For this review, take the finished solid that the model builds, in its own axes (mm). Face numbers are marked on the shaded views. A direction names the side the tool comes from. Coordinates: 2 decimals unless noted, no trailing zeros. Write each loop counter-clockwise with the first axis right and the second up, starting at its lowest first coordinate (ties: lowest second). Pieces come first, ordered by that corner, then holes. Notation, with made-up numbers: (82.25, 58.5) - (141.25, 58.5) arc R10 cw to (141.25, 62.5) - close; hole circle Ø1 at (-25.5, -30). An arc over 180 degrees is marked (long way). Use one line per item in the form item = value. Start each with the question number.
1) Mouldability with a two-part tool opening along Y and no side actions: class the marked faces 1, 2, 3 and 4 as pulls with the +Y half, pulls with the -Y half, needs draft (parallel to the pull), parting line crosses it, or undercut.
2) We need section C-C (y = -20). Give the boundary of the cut face in (x, z), plus the area to 3 significant figures.
3) Tool access review of the marked faces 5, 6, 7 and 8: name each direction out of +Z, -Z, +X, -X, +Y, -Y from which nothing blocks a thin tool from reaching the whole face with its end or side.
4) Insertion check: P1, Ø3, axis at x = 9, y = 5, coming from the -Z side; P2, Ø3, axis at y = 2, z = -2, coming from the +X side; P3, Ø1, axis at y = 11.5, z = 1, coming from the -X side; P4, Ø3, axis at x = -0.84, y = -12.32, coming from the +Z side. Each pin has a flat end and moves straight along its axis. Give the tip position at first contact, or say it passes through.
5) We need section A-A (z = 1). Count the separate pieces of the cut face and the enclosed holes in it, plus the area to 3 significant figures.
6) For L1, parallel to Y at x = -1.5, z = -3.75; L2, parallel to Y at x = 1, z = -1.5; L3, parallel to Z at x = 12.5, y = -3.5, list the stretches that pass through material, from the lowest coordinate up. Write a range as from..to.
7) We need section D-D (x = 12). Give the boundary of the cut face in (y, z).
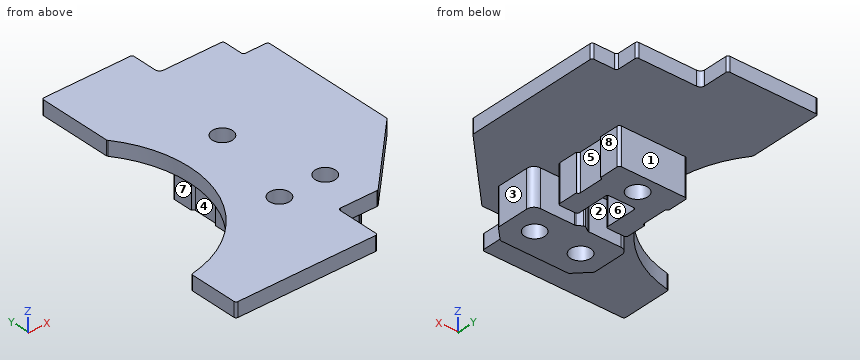
Autodesk Inventor part; units mm, degrees
ref_plane "Work Plane1" through (-17.3538, -25.3153, -5.1) normal (0, 0, 1) x (1, 0, 0)
ref_plane "Work Plane2" through (282.7327, 0, 0) normal (0, 0, 1) x (1, 0, 0)
ref_plane "YZ Plane" through (0, 0, 0) normal (1, 0, 0) x (0, 1, 0)
ref_plane "Work Plane1" through (-17.3538, -25.3153, -5.1) normal (0, 0, 1) x (1, 0, 0)
sketch "holes" plane through (0, 0, 0) normal (0, 0, 1) x (1, 0, 0)
  arc A0 (17.3538, 10.1647) -> (17.0538, 10.4647) centre (17.0538, 10.1647) ccw
  line L0 (17.0538, 10.4647) -> (14.2323, 10.4647)
  arc A1 (13.9323, 10.7647) -> (14.2323, 10.4647) centre (14.2323, 10.7647) ccw
  line L1 (13.9323, 10.7647) -> (13.9323, 13.3588)
  arc A2 (13.9323, 13.3588) -> (13.6323, 13.6588) centre (13.6323, 13.3588) ccw
  line L2 (13.6323, 13.6588) -> (5.6606, 13.6588)
  arc A3 (5.0636, 14.2558) -> (5.6606, 13.6588) centre (5.6606, 14.2558) ccw
  line L3 (5.0636, 14.2558) -> (5.0636, 17.6129)
  arc A4 (5.0636, 17.6129) -> (4.7636, 17.9129) centre (4.7636, 17.6129) ccw
  line L4 (4.7636, 17.9129) -> (-1.9383, 17.9129)
  arc A5 (-2.2383, 18.2129) -> (-1.9383, 17.9129) centre (-1.9383, 18.2129) ccw
  line L5 (-2.2383, 18.2129) -> (-2.2383, 18.3742)
  arc A6 (-2.2383, 18.3742) -> (-2.5383, 18.6742) centre (-2.5383, 18.3742) ccw
  line L6 (-2.5383, 18.6742) -> (-3.5364, 18.6742)
  arc A7 (-3.8364, 18.9742) -> (-3.5364, 18.6742) centre (-3.5364, 18.9742) ccw
  line L7 (-3.8364, 18.9742) -> (-3.8364, 19.9671)
  arc A8 (-3.8364, 19.9671) -> (-4.1364, 20.2671) centre (-4.1364, 19.9671) ccw
  line L8 (-4.1364, 20.2671) -> (-5.1364, 20.2671)
  arc A9 (-5.4364, 20.5671) -> (-5.1364, 20.2671) centre (-5.1364, 20.5671) ccw
  line L9 (-5.4364, 20.5671) -> (-5.4364, 24.1018)
  arc A10 (-5.4364, 24.1018) -> (-5.7364, 24.4018) centre (-5.7364, 24.1018) ccw
  line L10 (-5.7364, 24.4018) -> (-7.1364, 24.4018)
  arc A11 (-7.1364, 24.4018) -> (-7.4364, 24.1018) centre (-7.1364, 24.1018) ccw
  line L11 (-7.4364, 24.1018) -> (-7.4364, 7.6483)
  arc A12 (-7.4364, 7.6483) -> (-7.3759, 7.4677) centre (-7.1364, 7.6483) ccw
  arc A13 (-17.115, -17.2892) -> (-7.3759, 7.4677) centre (-19.8297, -1.9272) ccw
  arc A14 (-17.115, -17.2892) -> (-17.3538, -17.5116) centre (-17.0628, -17.5846) ccw
  line L12 (-17.3538, -17.5116) -> (-17.3538, -24.1018)
  arc A15 (-17.3538, -24.1018) -> (-17.0538, -24.4018) centre (-17.0538, -24.1018) ccw
  line L13 (-17.0538, -24.4018) -> (1.9557, -24.4018)
  arc A16 (1.9557, -24.4018) -> (2.2557, -24.1018) centre (1.9557, -24.1018) ccw
  line L14 (2.2557, -24.1018) -> (2.2557, -18.3961)
  arc A17 (2.5557, -18.0961) -> (2.2557, -18.3961) centre (2.5557, -18.3961) ccw
  line L15 (2.5557, -18.0961) -> (7.6549, -18.0961)
  arc A18 (7.6549, -18.0961) -> (7.8673, -18.008) centre (7.6549, -17.7961) ccw
  line L16 (7.8673, -18.008) -> (17.2662, -8.5819)
  arc A19 (17.2662, -8.5819) -> (17.3538, -8.3701) centre (17.0538, -8.3701) ccw
  line L17 (17.3538, -8.3701) -> (17.3538, 10.1647)
  arc A20 (1.196, -8.6701) -> (1.3547, -8.6247) centre (1.196, -8.3701) ccw
  line L18 (1.3547, -8.6247) -> (2.0283, -8.2049)
  arc A21 (2.3456, -8.2049) -> (2.0283, -8.2049) centre (2.187, -8.4595) ccw
  line L19 (2.3456, -8.2049) -> (3.0192, -8.6247)
  arc A22 (3.0192, -8.6247) -> (3.1779, -8.6701) centre (3.1779, -8.3701) ccw
  line L20 (3.1779, -8.6701) -> (7.8974, -8.6701)
  arc A23 (8.8974, -9.6701) -> (7.8974, -8.6701) centre (7.8974, -9.6701) ccw
  line L21 (8.8974, -9.6701) -> (8.8974, -14.0729)
  arc A24 (8.8069, -14.2875) -> (8.8974, -14.0729) centre (8.5974, -14.0729) ccw
  line L22 (8.8069, -14.2875) -> (7.1705, -15.8848)
  arc A25 (6.9609, -15.9701) -> (7.1705, -15.8848) centre (6.9609, -15.6701) ccw
  line L23 (6.9609, -15.9701) -> (-2.2459, -15.9701)
  arc A26 (-2.4611, -15.8791) -> (-2.2459, -15.9701) centre (-2.2459, -15.6701) ccw
  line L24 (-2.4611, -15.8791) -> (-4.1564, -14.1338)
  arc A27 (-4.2412, -13.9247) -> (-4.1564, -14.1338) centre (-3.9412, -13.9247) ccw
  line L25 (-4.2412, -13.9247) -> (-4.2412, -9.6701)
  arc A28 (-3.2412, -8.6701) -> (-4.2412, -9.6701) centre (-3.2412, -9.6701) ccw
  line L26 (-3.2412, -8.6701) -> (1.196, -8.6701)
  arc A29 (4.2967, -2.4382) -> (3.9967, -2.1382) centre (3.9967, -2.4382) ccw
  line L27 (3.9967, -2.1382) -> (0.6538, -2.1382)
  arc A30 (0.6538, -2.1382) -> (0.3538, -2.4382) centre (0.6538, -2.4382) ccw
  line L28 (0.3538, -2.4382) -> (0.3538, -6.5942)
  arc A31 (0.0538, -6.8942) -> (0.3538, -6.5942) centre (0.0538, -6.5942) ccw
  line L29 (0.0538, -6.8942) -> (-2.1438, -6.8942)
  arc A32 (-2.4438, -6.5942) -> (-2.1438, -6.8942) centre (-2.1438, -6.5942) ccw
  line L30 (-2.4438, -6.5942) -> (-2.4438, -3.9753)
  arc A33 (-2.4438, -3.9753) -> (-2.1438, -3.6753) centre (-2.4438, -3.6753) ccw
  line L31 (-2.1438, -3.6753) -> (-2.1438, -0.4348)
  arc A34 (-2.1438, -0.4348) -> (-2.4438, -0.1348) centre (-2.4438, -0.4348) ccw
  line L32 (-2.4438, -0.1348) -> (-2.4438, 2.5284)
  arc A35 (-2.1438, 2.8284) -> (-2.4438, 2.5284) centre (-2.1438, 2.5284) ccw
  line L33 (-2.1438, 2.8284) -> (6.6827, 2.8284)
  arc A36 (6.9827, 2.5284) -> (6.6827, 2.8284) centre (6.6827, 2.5284) ccw
  line L34 (6.9827, 2.5284) -> (6.9827, -0.1348)
  arc A37 (6.9827, -0.1348) -> (6.6827, -0.4348) centre (6.9827, -0.4348) ccw
  line L35 (6.6827, -0.4348) -> (6.6827, -3.6753)
  arc A38 (6.6827, -3.6753) -> (6.9827, -3.9753) centre (6.9827, -3.6753) ccw
  line L36 (6.9827, -3.9753) -> (6.9827, -6.5942)
  arc A39 (6.6827, -6.8942) -> (6.9827, -6.5942) centre (6.6827, -6.5942) ccw
  line L37 (6.6827, -6.8942) -> (4.5967, -6.8942)
  arc A40 (4.2967, -6.5942) -> (4.5967, -6.8942) centre (4.5967, -6.5942) ccw
  line L38 (4.2967, -6.5942) -> (4.2967, -2.4382)
  circle A41 centre (2.2695, 0.3451) radius 1.4
  circle A42 centre (5.4974, -12.3201) radius 1.4
  circle A43 centre (-0.8412, -12.3201) radius 1.4
  line L39 (-7.1364, 17.9129) -> (4.7636, 17.9129)
  arc A44 (-7.1364, 17.9129) -> (-7.4364, 17.6129) centre (-7.1364, 17.6129) ccw
  line L40 (-7.4364, 7.6483) -> (-7.4364, 17.6129)
  point P0 (0, 0)
extrude "Extrusion1" add sketch "holes" against normal up to surface (5.1 mm away) contours A20 L18 A21 L19 A22 L20 A23 L21 A24 L22 A25 L23 A26 L24 A27 L25 A28 L26 | A29 L27 A30 L28 A31 L29 A32 L30 A33 L31 A34 L32 A35 L33 A36 L34 A37 L35 A38 L36 A39 L37 A40 L38
ref_plane "Work Plane2" through (282.7327, 0, 0) normal (0, 0, 1) x (1, 0, 0)
sketch "plate" plane through (0, 0, 0) normal (0, 0, 1) x (1, 0, 0)
  arc A0 (17.3538, 10.1647) -> (17.0538, 10.4647) centre (17.0538, 10.1647) ccw
  line L0 (17.0538, 10.4647) -> (14.2323, 10.4647)
  arc A1 (13.9323, 10.7647) -> (14.2323, 10.4647) centre (14.2323, 10.7647) ccw
  line L1 (13.9323, 10.7647) -> (13.9323, 13.3588)
  arc A2 (13.9323, 13.3588) -> (13.6323, 13.6588) centre (13.6323, 13.3588) ccw
  line L2 (13.6323, 13.6588) -> (5.6606, 13.6588)
  arc A3 (5.0636, 14.2558) -> (5.6606, 13.6588) centre (5.6606, 14.2558) ccw
  line L3 (5.0636, 14.2558) -> (5.0636, 17.6129)
  arc A4 (5.0636, 17.6129) -> (4.7636, 17.9129) centre (4.7636, 17.6129) ccw
  line L4 (4.7636, 17.9129) -> (-1.9383, 17.9129)
  arc A5 (-2.2383, 18.2129) -> (-1.9383, 17.9129) centre (-1.9383, 18.2129) ccw
  line L5 (-2.2383, 18.2129) -> (-2.2383, 18.3742)
  arc A6 (-2.2383, 18.3742) -> (-2.5383, 18.6742) centre (-2.5383, 18.3742) ccw
  line L6 (-2.5383, 18.6742) -> (-3.5364, 18.6742)
  arc A7 (-3.8364, 18.9742) -> (-3.5364, 18.6742) centre (-3.5364, 18.9742) ccw
  line L7 (-3.8364, 18.9742) -> (-3.8364, 19.9671)
  arc A8 (-3.8364, 19.9671) -> (-4.1364, 20.2671) centre (-4.1364, 19.9671) ccw
  line L8 (-4.1364, 20.2671) -> (-5.1364, 20.2671)
  arc A9 (-5.4364, 20.5671) -> (-5.1364, 20.2671) centre (-5.1364, 20.5671) ccw
  line L9 (-5.4364, 20.5671) -> (-5.4364, 24.1018)
  arc A10 (-5.4364, 24.1018) -> (-5.7364, 24.4018) centre (-5.7364, 24.1018) ccw
  line L10 (-5.7364, 24.4018) -> (-7.1364, 24.4018)
  arc A11 (-7.1364, 24.4018) -> (-7.4364, 24.1018) centre (-7.1364, 24.1018) ccw
  line L11 (-7.4364, 24.1018) -> (-7.4364, 7.6483)
  arc A12 (-7.4364, 7.6483) -> (-7.3759, 7.4677) centre (-7.1364, 7.6483) ccw
  arc A13 (-17.115, -17.2892) -> (-7.3759, 7.4677) centre (-19.8297, -1.9272) ccw
  arc A14 (-17.115, -17.2892) -> (-17.3538, -17.5116) centre (-17.0628, -17.5846) ccw
  line L12 (-17.3538, -17.5116) -> (-17.3538, -24.1018)
  arc A15 (-17.3538, -24.1018) -> (-17.0538, -24.4018) centre (-17.0538, -24.1018) ccw
  line L13 (-17.0538, -24.4018) -> (1.9557, -24.4018)
  arc A16 (1.9557, -24.4018) -> (2.2557, -24.1018) centre (1.9557, -24.1018) ccw
  line L14 (2.2557, -24.1018) -> (2.2557, -18.3961)
  arc A17 (2.5557, -18.0961) -> (2.2557, -18.3961) centre (2.5557, -18.3961) ccw
  line L15 (2.5557, -18.0961) -> (7.6549, -18.0961)
  arc A18 (7.6549, -18.0961) -> (7.8673, -18.008) centre (7.6549, -17.7961) ccw
  line L16 (7.8673, -18.008) -> (17.2662, -8.5819)
  arc A19 (17.2662, -8.5819) -> (17.3538, -8.3701) centre (17.0538, -8.3701) ccw
  line L17 (17.3538, -8.3701) -> (17.3538, 10.1647)
  arc A20 (1.196, -8.6701) -> (1.3547, -8.6247) centre (1.196, -8.3701) ccw
  line L18 (1.3547, -8.6247) -> (2.0283, -8.2049)
  arc A21 (2.3456, -8.2049) -> (2.0283, -8.2049) centre (2.187, -8.4595) ccw
  line L19 (2.3456, -8.2049) -> (3.0192, -8.6247)
  arc A22 (3.0192, -8.6247) -> (3.1779, -8.6701) centre (3.1779, -8.3701) ccw
  line L20 (3.1779, -8.6701) -> (7.8974, -8.6701)
  arc A23 (8.8974, -9.6701) -> (7.8974, -8.6701) centre (7.8974, -9.6701) ccw
  line L21 (8.8974, -9.6701) -> (8.8974, -14.0729)
  arc A24 (8.8069, -14.2875) -> (8.8974, -14.0729) centre (8.5974, -14.0729) ccw
  line L22 (8.8069, -14.2875) -> (7.1705, -15.8848)
  arc A25 (6.9609, -15.9701) -> (7.1705, -15.8848) centre (6.9609, -15.6701) ccw
  line L23 (6.9609, -15.9701) -> (-2.2459, -15.9701)
  arc A26 (-2.4611, -15.8791) -> (-2.2459, -15.9701) centre (-2.2459, -15.6701) ccw
  line L24 (-2.4611, -15.8791) -> (-4.1564, -14.1338)
  arc A27 (-4.2412, -13.9247) -> (-4.1564, -14.1338) centre (-3.9412, -13.9247) ccw
  line L25 (-4.2412, -13.9247) -> (-4.2412, -9.6701)
  arc A28 (-3.2412, -8.6701) -> (-4.2412, -9.6701) centre (-3.2412, -9.6701) ccw
  line L26 (-3.2412, -8.6701) -> (1.196, -8.6701)
  arc A29 (4.2967, -2.4382) -> (3.9967, -2.1382) centre (3.9967, -2.4382) ccw
  line L27 (3.9967, -2.1382) -> (0.6538, -2.1382)
  arc A30 (0.6538, -2.1382) -> (0.3538, -2.4382) centre (0.6538, -2.4382) ccw
  line L28 (0.3538, -2.4382) -> (0.3538, -6.5942)
  arc A31 (0.0538, -6.8942) -> (0.3538, -6.5942) centre (0.0538, -6.5942) ccw
  line L29 (0.0538, -6.8942) -> (-2.1438, -6.8942)
  arc A32 (-2.4438, -6.5942) -> (-2.1438, -6.8942) centre (-2.1438, -6.5942) ccw
  line L30 (-2.4438, -6.5942) -> (-2.4438, -3.9753)
  arc A33 (-2.4438, -3.9753) -> (-2.1438, -3.6753) centre (-2.4438, -3.6753) ccw
  line L31 (-2.1438, -3.6753) -> (-2.1438, -0.4348)
  arc A34 (-2.1438, -0.4348) -> (-2.4438, -0.1348) centre (-2.4438, -0.4348) ccw
  line L32 (-2.4438, -0.1348) -> (-2.4438, 2.5284)
  arc A35 (-2.1438, 2.8284) -> (-2.4438, 2.5284) centre (-2.1438, 2.5284) ccw
  line L33 (-2.1438, 2.8284) -> (6.6827, 2.8284)
  arc A36 (6.9827, 2.5284) -> (6.6827, 2.8284) centre (6.6827, 2.5284) ccw
  line L34 (6.9827, 2.5284) -> (6.9827, -0.1348)
  arc A37 (6.9827, -0.1348) -> (6.6827, -0.4348) centre (6.9827, -0.4348) ccw
  line L35 (6.6827, -0.4348) -> (6.6827, -3.6753)
  arc A38 (6.6827, -3.6753) -> (6.9827, -3.9753) centre (6.9827, -3.6753) ccw
  line L36 (6.9827, -3.9753) -> (6.9827, -6.5942)
  arc A39 (6.6827, -6.8942) -> (6.9827, -6.5942) centre (6.6827, -6.5942) ccw
  line L37 (6.6827, -6.8942) -> (4.5967, -6.8942)
  arc A40 (4.2967, -6.5942) -> (4.5967, -6.8942) centre (4.5967, -6.5942) ccw
  line L38 (4.2967, -6.5942) -> (4.2967, -2.4382)
  arc A41 (-7.1364, 17.9129) -> (-7.4364, 17.6129) centre (-7.1364, 17.6129) ccw
  line L39 (-7.1364, 17.9129) -> (4.7636, 17.9129)
  circle A42 centre (2.2695, 0.3451) radius 1.4
  circle A43 centre (5.4974, -12.3201) radius 1.4
  circle A44 centre (-0.8412, -12.3201) radius 1.4
  point P0 (0, 0)
extrude "Extrusion2" add sketch "plate" along normal blind 2 contours L17 A19 L16 A18 L15 A17 L14 A16 L13 A15 L12 A14 A13 A12 L11 A41 L39 L4 A4 L3 A3 L2 A2 L1 A1 L0 A0 | A20 L18 A21 L19 A22 L20 A23 L21 A24 L22 A25 L23 A26 L24 A27 L25 A28 L26 | A29 L27 A30 L28 A31 L29 A32 L30 A33 L31 A34 L32 A35 L33 A36 L34 A37 L35 A38 L36 A39 L37 A40 L38
properties part number "mount_carriage_bottom"
Determined:
q1.face_1 = pulls with the +Y half
q1.face_2 = undercut
q1.face_3 = needs draft
q1.face_4 = undercut
q2.outline = (-17.35, 0) - (2.26, 0) - (2.26, 2) - (-17.35, 2) - close
q2.area = 39.2 mm²
q3.face_5 = -Z, +X
q3.face_6 = -Z
q3.face_7 = -Z, -X, +Y
q3.face_8 = -Z, +X, +Y
q4.P1 = 0
q4.P2 = 6.98
q4.P3 = -7.44
q4.P4 = 2
q5.separate_pieces = 1
q5.enclosed_holes = 3
q5.area = 876 mm²
q6.L1 = -15.97..-13.56, -11.08..-8.67, -6.89..2.83
q6.L2 = -15.97..-8.67, -2.14..-0.25, 0.94..2.83
q6.L3 = 0..2
q7.outline = (-13.86, 0) - (13.66, 0) - (13.66, 2) - (-13.86, 2) - close
